```python
from build123d import *

# Parameters (mm, degrees)
SKETCH1_W           = 170
SKETCH1_H           = 50
BOSS_EXTRUDE1_DEPTH = 2
SKETCH2_W           = 2
SKETCH2_H           = 50
BOSS_EXTRUDE2_DEPTH = 10
SKETCH3_W           = 150
SKETCH3_H           = 2
BOSS_EXTRUDE3_DEPTH = 10
SKETCH4_W           = 60
SKETCH4_H           = 50
CUT_EXTRUDE2_DEPTH  = 13
BOSS_EXTRUDE5_DEPTH = 12
BOSS_EXTRUDE7_DEPTH = 2
SKETCH8_W           = 4
SKETCH8_H           = 20
CUT_EXTRUDE3_DEPTH  = 2


with BuildPart() as part:
    # Sketch1 → Boss-Extrude1 (new body)
    with BuildSketch(Plane(origin=(0, 0, 0), x_dir=(1, 0, 0), z_dir=(0, 1, 0))):
        with Locations((15.5, 15.5)):
            Rectangle(SKETCH1_W, SKETCH1_H)
        with BuildLine():
            Line((5, 32.75), (-5, 32.75))
            ThreePointArc((-5, 32.75), (-6.75, 31), (-5, 29.25))
            Line((-5, 29.25), (5, 29.25))
            ThreePointArc((5, 29.25), (6.749999891, 31), (5, 32.75))
        make_face(mode=Mode.SUBTRACT)
        with BuildLine():
            Line((26, 29.25), (36, 29.25))
            ThreePointArc((36, 29.25), (37.75, 31), (36, 32.75))
            Line((36, 32.75), (26, 32.75))
            ThreePointArc((26, 32.75), (24.25, 31), (26, 29.25))
        make_face(mode=Mode.SUBTRACT)
        with BuildLine():
            Line((-5, 1.75), (5, 1.75))
            ThreePointArc((5, 1.75), (6.75, 0), (5, -1.75))
            Line((5, -1.75), (-5, -1.75))
            ThreePointArc((-5, -1.75), (-6.75, 0), (-5, 1.75))
        make_face(mode=Mode.SUBTRACT)
        with BuildLine():
            Line((26, -1.75), (36, -1.75))
            ThreePointArc((36, -1.75), (37.75, 0), (36, 1.75))
            Line((36, 1.75), (26, 1.75))
            ThreePointArc((26, 1.75), (24.25, 0), (26, -1.75))
        make_face(mode=Mode.SUBTRACT)
        with BuildLine():
            Line((10.5, 27), (20.5, 27))
            ThreePointArc((20.5, 27), (32, 15.5), (20.5, 4))
            Line((20.5, 4), (10.5, 4))
            ThreePointArc((10.5, 4), (-1, 15.5), (10.5, 27))
        make_face(mode=Mode.SUBTRACT)
    extrude(amount=BOSS_EXTRUDE1_DEPTH)

    # Sketch2 → Boss-Extrude2 (add)
    with BuildSketch(Plane(origin=(0, 0, 0), x_dir=(-1, 0, 0), z_dir=(0, -1, 0))):
        with Locations((60.5, 15.5)):
            Rectangle(SKETCH2_W, SKETCH2_H)
        with Locations((-91.5, 15.5)):
            Rectangle(SKETCH2_W, SKETCH2_H)
    extrude(amount=BOSS_EXTRUDE2_DEPTH)

    # Sketch3 → Boss-Extrude3 (add)
    with BuildSketch(Plane(origin=(0, 0, 0), x_dir=(-1, 0, 0), z_dir=(0, -1, 0))):
        with Locations((-15.5, 39.5)):
            Rectangle(SKETCH3_W, SKETCH3_H)
        with Locations((-15.5, -8.5)):
            Rectangle(SKETCH3_W, SKETCH3_H)
    extrude(amount=BOSS_EXTRUDE3_DEPTH)

    # Sketch4 → Cut-Extrude2 (cut, through all)
    with BuildSketch(Plane(origin=(0, 2, 0), x_dir=(1, 0, 0), z_dir=(0, 1, 0))):
        with Locations((-39.5, 15.5)):
            Rectangle(SKETCH4_W, SKETCH4_H)
    cut_extrude2 = extrude(amount=-CUT_EXTRUDE2_DEPTH, mode=Mode.SUBTRACT)

    # Mirror1: Cut-Extrude2 across plane
    add(cut_extrude2.mirror(Plane.ZY.offset(-15.5)), mode=Mode.SUBTRACT)

    # Sketch5 → Boss-Extrude5 (add)
    with BuildSketch(Plane(origin=(0, 2, 0), x_dir=(1, 0, 0), z_dir=(0, 1, 0))):
        Polygon((40.5, 40.5), (90.5, 45.5), (90.5, -14.5), (40.5, -9.5), (40.5, -7.690024876), (40.5, 38.5), align=None)
        Polygon((42.5, 38.690024876), (68.491666638, 16.5), (88.5, 16.5), (88.5, 18.080254606), (88.5, 43.290024876), align=None, mode=Mode.SUBTRACT)
        Polygon((88.5, 14.5), (68.491666638, 14.5), (42.5, -7.690024876), (88.5, -12.290024876), align=None, mode=Mode.SUBTRACT)
        Polygon((66.582731952, 15.5), (42.5, 36.060298366), (42.5, -5.060298366), align=None, mode=Mode.SUBTRACT)
    boss_extrude5 = extrude(amount=-BOSS_EXTRUDE5_DEPTH)

    # Sketch7 → Boss-Extrude7 (add)
    with BuildSketch(Plane(origin=(0, 2, 0), x_dir=(1, 0, 0), z_dir=(0, 1, 0))):
        Polygon((90.5, -14.5), (105.5, -15.740832862), (105.5, 46.740832862), (90.5, 45.5), align=None)
    boss_extrude7 = extrude(amount=-BOSS_EXTRUDE7_DEPTH)

    # Sketch8 → Cut-Extrude3 (cut)
    with BuildSketch(Plane(origin=(0, 2, 0), x_dir=(1, 0, 0), z_dir=(0, 1, 0))):
        with Locations((97, 0.5)):
            Rectangle(SKETCH8_W, SKETCH8_H)
        with Locations((97, 30.5)):
            Rectangle(SKETCH8_W, SKETCH8_H)
    cut_extrude3 = extrude(amount=-CUT_EXTRUDE3_DEPTH, mode=Mode.SUBTRACT)

    # Mirror2: Boss-Extrude5, Boss-Extrude7, Cut-Extrude3 across plane
    add(boss_extrude5.mirror(Plane.ZY.offset(-15.5)))
    add(boss_extrude7.mirror(Plane.ZY.offset(-15.5)))
    add(cut_extrude3.mirror(Plane.ZY.offset(-15.5)), mode=Mode.SUBTRACT)


solid = part.part
```
Source: CAD feature listing. Evaluate the final solid. Frame: model axes, mm. A direction names the side the tool comes from. Coordinates: 2 decimals unless noted, no trailing zeros. Write each loop counter-clockwise with the first axis right and the second up, starting at its lowest first coordinate (ties: lowest second). Pieces come first, ordered by that corner, then holes. Notation, with made-up numbers: (-21, 80) - (13, 80) arc R26 ccw to (13, 96) - close; hole circle Ø2 at (-5.5, 34.25). An arc over 180 degrees is marked (long way). Answer as a JSON object with one key per item and string values.
Q1. Section query A-A, the plane x = 16.5. Output: boundary loops of the cut face in (y, z), plus the area to 3 significant figures.
Ans:
{"outline": "(-10, -40.5) - (2, -40.5) - (2, -27) - (0, -27) - (0, -38.5) - (-10, -38.5) - close; (-10, 7.5) - (0, 7.5) - (0, -4) - (2, -4) - (2, 9.5) - (-10, 9.5) - close", "area": "94.0 mm2"}
Q2. Set-up query: faces 4 (the flat face through (-67, 0, -16)), 5 (the flat face through (-34.822, -3.916, -41.022)), 6 (the flat face through (65.85, -3.916, 12.035)), 7 (the flat face through (65.15, -3.916, -42.965)). Return all of +Z, -Z, +X, -X, +Y, -Y with unobstructed straight access to the full face (end or side cutting, diameter ignored); none if empty.
Ans:
{"face 4": "+Z, -Z, -X, -Y", "face 5": "+Y, -Y", "face 6": "+Z, +Y, -Y", "face 7": "-Z, +Y, -Y"}
Q3. Section query B-B, the plane y = -2.5. State how many separate pieces and enclosed holes the cut face has, plus the area to 3 significant figures.
Ans:
{"separate pieces": "1", "enclosed holes": "7", "area": "1,360 mm2"}
Q4. Material intervals for line 1 (Z direction, x = 7.5, y = -5.5); line 2 (X direction, y = -8.75, z = -28); line 3 (Z direction, x = -13, y = -8), sorted ascending. Write a range as [from, to].
Ans:
{"line 1": "z = [-40.5, -38.5], [7.5, 9.5]", "line 2": "x = [-59.5, -57.5], [-24.02, -20.94], [-11.5, -9.5], [40.5, 42.5], [51.94, 55.02], [88.5, 90.5]", "line 3": "z = [-40.85, -38.84], [-37.41, -34.78], [3.78, 6.41], [7.84, 9.85]"}
Q5. Section query D-D, the plane x = 54. Output: boundary loops of the cut face in (y, z).
Ans:
{"outline": "(-10, -41.85) - (2, -41.85) - (2, -39.84) - (-10, -39.84) - close; (-10, -28.87) - (2, -28.87) - (2, -26.24) - (-10, -26.24) - close; (-10, -4.76) - (2, -4.76) - (2, -2.13) - (-10, -2.13) - close; (-10, 8.84) - (2, 8.84) - (2, 10.85) - (-10, 10.85) - close"}
Q6. First-contact query: pin 1 Ø0.6 at (x, y) = (1, 1) entering from +Z; pin 2 Ø2 at (x, y) = (14.5, 1) entering from -Z; pin 3 Ø6 at (y, z) = (-7, -29) entering from -X; pin 4 Ø6 at (y, z) = (-1.5, -32.5) entering from +X. Flat tips, straight axial feed; report the tip coordinate or a pass-through.
Ans:
{"pin 1": "stops at z = 9.5", "pin 2": "stops at z = -40.5", "pin 3": "stops at x = -59.5", "pin 4": "stops at x = 105.5"}
Q7. Section query C-C, the plane x = -41. Output: boundary loops of the cut face in (y, z).
Ans:
{"outline": "(-10, -43.65) - (2, -43.65) - (2, -41.64) - (-10, -41.64) - close; (-10, -16.5) - (2, -16.5) - (2, -14.5) - (-10, -14.5) - close; (-10, 10.64) - (2, 10.64) - (2, 12.65) - (-10, 12.65) - close"}
Q8. Draft query along Y for faces 1 (the flat face through (4, 0, -26)), 2 (the flat face through (-59.5, -5, -16)), 3 (the flat face through (-3, 2, -16)). Return one class per face: released by +Y, released by -Y, zero draft, split by the parting line, or undercut.
Ans:
{"face 1": "released by -Y", "face 2": "zero draft", "face 3": "released by +Y"}
